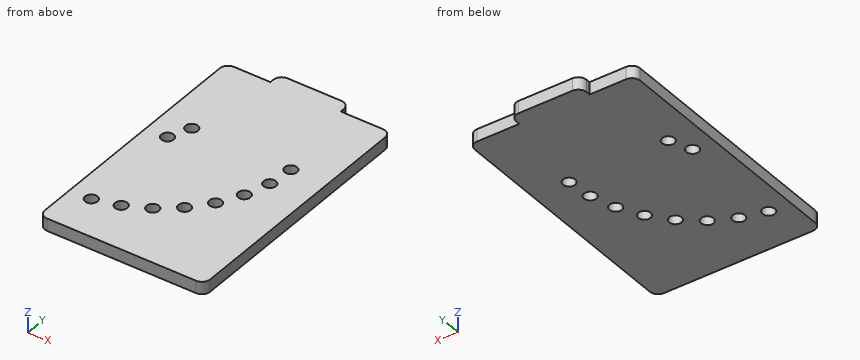
```python
from build123d import *

# Parameters (mm, degrees)
SKETCH_1_R      = 1.5
SKETCH_1_W      = 17
SKETCH_1_H      = 3
EXTRUDE_1_DEPTH = 3
FILLET_1_R      = 2
FILLET_2_R      = 2


with BuildPart() as part:
    # 草图1 → 凸台-拉伸1 (new body)
    # profile 1 of 5: a face of its own
    with BuildSketch(Plane.XY):
        with BuildLine():
            Line((0, 10), (0, 7))
            ThreePointArc((0, 7), (24.26790473, 17.05209527), (34.32, 41.32))
            Line((34.32, 41.32), (34.32, 63))
            Line((34.32, 63), (4.32, 63))
            Line((4.32, 63), (4.32, 41.32))
            ThreePointArc((4.32, 41.32), (3.054701295, 38.265298705), (0, 37))
            Line((0, 37), (0, 34))
            Line((0, 34), (0, 22))
            Line((0, 22), (0, 10))
        make_face()
        with Locations((5.176021638, 10.430662034)):
            Circle(SKETCH_1_R, mode=Mode.SUBTRACT)
        with Locations((11.229544899, 12.082357801)):
            Circle(SKETCH_1_R, mode=Mode.SUBTRACT)
        with Locations((16.832334664, 14.907599318)):
            Circle(SKETCH_1_R, mode=Mode.SUBTRACT)
        with Locations((21.759505147, 18.792986533)):
            Circle(SKETCH_1_R, mode=Mode.SUBTRACT)
        with Locations((25.813288692, 23.582567072)):
            Circle(SKETCH_1_R, mode=Mode.SUBTRACT)
        with Locations((28.830973806, 29.08409589)):
            Circle(SKETCH_1_R, mode=Mode.SUBTRACT)
        with Locations((30.691436099, 35.076751631)):
            Circle(SKETCH_1_R, mode=Mode.SUBTRACT)
        with Locations((31.32, 41.32)):
            Circle(SKETCH_1_R, mode=Mode.SUBTRACT)
        with Locations((7.32, 41.32)):
            Circle(SKETCH_1_R, mode=Mode.SUBTRACT)
        with Locations((5.176021638, 36.143978362)):
            Circle(SKETCH_1_R, mode=Mode.SUBTRACT)
    # profile 2 of 5: a face of its own
    with BuildSketch(Plane.XY):
        with BuildLine():
            Line((0, 41.32), (0, 37))
            ThreePointArc((0, 37), (3.054701295, 38.265298705), (4.32, 41.32))
            Line((4.32, 41.32), (4.32, 63))
            Line((4.32, 63), (0, 63))
            Line((0, 63), (0, 41.32))
        make_face()
    # profile 3 of 5: a face of its own
    with BuildSketch(Plane.XY):
        with BuildLine():
            ThreePointArc((0, 7), (24.26790473, 17.05209527), (34.32, 41.32))
            Line((34.32, 41.32), (34.32, 63))
            Line((34.32, 63), (40, 63))
            Line((40, 63), (40, 0))
            Line((40, 0), (0, 0))
            Line((0, 0), (0, 7))
        make_face()
    # profile 4 of 5: a face of its own
    with BuildSketch(Plane.XY):
        with Locations((19.32, 64.5)):
            Rectangle(SKETCH_1_W, SKETCH_1_H)
    # profile 5 of 5: a face of its own
    with BuildSketch(Plane.XY):
        with BuildLine():
            ThreePointArc((34.32, 41.32), (24.26790473, 17.05209527), (0, 7))
            Line((0, 7), (0, 0))
            Line((0, 0), (40, 0))
            Line((40, 0), (40, 63))
            Line((40, 63), (34.32, 63))
            Line((34.32, 63), (34.32, 41.32))
        make_face()
    extrude(amount=EXTRUDE_1_DEPTH)

    # 圆角1
    fillet_1_edges = [part.edges().sort_by_distance(p)[0] for p in [
        (40, 63, 1.5),
        (40, 0, 1.5),
        (0, 0, 1.5),
        (0, 63, 1.5),
    ]]
    fillet(fillet_1_edges, radius=FILLET_1_R)

    # 圆角2
    fillet_2_edges = [part.edges().sort_by_distance(p)[0] for p in [
        (10.82, 66, 1.5),
        (27.82, 66, 1.5),
    ]]
    fillet(fillet_2_edges, radius=FILLET_2_R)


solid = part.part
```
Check sheet for the modelled part. Datum: model origin and axes. Units: mm. Round coordinates to 2 decimals unless told otherwise and drop trailing zeros. Order: outer loops, then holes, each group sorted by start corner. A loop starts at its lowest first (then second) coordinate and runs counter-clockwise, first axis right, second up. Notation, with made-up numbers: (57.5, 30) -> (70.5, 30) arc R30 cw to (70.5, 55) -> close; hole circle Ø11 at (-26.5, -20). An arc over 180 degrees is marked (long way). Use CSV: the item, a comma, the result in double quotes.
(1) Depth check by flat-ended pin: pin 1 (5 mm diameter, centred on x = 11.23, y = 12.08, fed in from +Z); pin 2 (1 mm diameter, centred on x = 5.5, z = 1, fed in from +Y); pin 3 (0.5 mm diameter, centred on y = 63.5, z = 2, fed in from +X). Enter the tip coordinate at first touch or a pass-through.
Worked out:
pin 1,"z = 3"
pin 2,"y = 63"
pin 3,"x = 27.82"
(2) Cross-section at B-B (y = 41.32). Record the boundary of the cut face in (x, z).
Worked out:
outline,"(0, 0) -> (5.82, 0) -> (5.82, 3) -> (0, 3) -> close; (8.82, 0) -> (29.82, 0) -> (29.82, 3) -> (8.82, 3) -> close; (32.82, 0) -> (40, 0) -> (40, 3) -> (32.82, 3) -> close"
(3) Cross-section at C-C (x = 31.32). Record the boundary of the cut face in (y, z).
Worked out:
outline,"(0, 0) -> (33.71, 0) -> (33.71, 3) -> (0, 3) -> close; (36.44, 0) -> (39.82, 0) -> (39.82, 3) -> (36.44, 3) -> close; (42.82, 0) -> (63, 0) -> (63, 3) -> (42.82, 3) -> close"
(4) Cross-section at D-D (z = 1). Count the separate pieces of the cut face and the enclosed holes in it, and give its area (3 significant figures).
Worked out:
separate pieces,"1"
enclosed holes,"10"
area,"2,500 mm²"
(5) Material ranges on line 1 along Y through (x, z) = (5, 2.65); line 2 along Y through (x, z) = (29, 0.2); line 3 along Y through (x, z) = (6.5, 0.9), recorded low to high. Write a range as from..to.
Worked out:
line 1,"0..8.94, 11.92..34.65, 37.63..63"
line 2,"0..27.59, 30.57..63"
line 3,"0..9.73, 11.14..35.44, 36.85..40.06, 42.58..63"
(6) Cross-section at A-A (x = 7.32). Record the boundary of the cut face in (y, z).
Worked out:
outline,"(0, 0) -> (39.82, 0) -> (39.82, 3) -> (0, 3) -> close; (42.82, 0) -> (63, 0) -> (63, 3) -> (42.82, 3) -> close"
